Autodesk Inventor part; units mm, degrees
ref_plane "YZ Plane" through (0, 0, 0) normal (1, 0, 0) x (0, 1, 0)
ref_plane "XZ Plane" through (0, 0, 0) normal (0, 1, 0) x (-1, 0, 0)
ref_plane "XY Plane" through (0, 0, 0) normal (0, 0, 1) x (1, 0, 0)
sketch "スケッチ1" plane through (0, 0, 0) normal (0, 0, 1) x (1, 0, 0)
  line L0 (0, 0) -> (15, 0)
  line L1 (15, 0) -> (15, 15)
  line L2 (15, 15) -> (0, 15)
  line L3 (0, 15) -> (0, 0)
  line L4 (1, 1) -> (14, 1)
  line L5 (14, 1) -> (14, 14)
  line L6 (14, 14) -> (1, 14)
  line L7 (1, 14) -> (1, 1)
  dimension "d0" = 15
  dimension "d1" = 15
  dimension "d2" = 13
  dimension "d3" = 13
  dimension "d4" = 1
  dimension "d5" = 1
extrude "押し出し1" add sketch "スケッチ1" along normal blind 46
sketch "スケッチ2" plane through (15, 0, 0) normal (1, 0, 0) x (0, 0, -1)
  circle A0 centre (-5, 7.5) radius 1.6
  line L0 (0, 0) -> (-46, 0)
  line L1 (0, 0) -> (0, 15)
  circle A1 centre (-41, 7.5) radius 1.6
  line L2 (-46, 0) -> (-46, 15)
  dimension "d8" = 3.2
  dimension "d9" = 7.5
  dimension "d10" = 5
  dimension "d11" = 3.2
  dimension "d12" = 5
hole "穴1" at (15, 7.5, 41) at (15, 7.5, 5) direction (-1, 0, 0) diameter 3.2 depth 15
sketch "スケッチ3" plane through (0, 15, 0) normal (0, 1, 0) x (1, 0, 0)
  circle A0 centre (7.5, -15) radius 1.6
  line L0 (15, 0) -> (15, -46)
  line L1 (15, 0) -> (0, 0)
  circle A1 centre (7.5, -31) radius 1.6
  line L2 (15, -46) -> (0, -46)
  dimension "d20" = 3.2
  dimension "d21" = 7.5
  dimension "d22" = 15
  dimension "d23" = 3.2
  dimension "d24" = 15
hole "穴2" at (7.5, 15, 31) at (7.5, 15, 15) direction (0, -1, 0) diameter 3.2 depth 15
equation "\"BendRadius\" = Thickness"
equation "\"BendReliefWidth\" = Thickness"
equation "\"BendReliefDepth\" = 0.5 * Thickness"
equation "\"CornerReliefSize\" = 4 * Thickness"
equation "\"MinimumRemnant\" = 2 * Thickness"
equation "\"TransitionRadius\" = BendRadius"
equation "\"JacobiRadiusSize\" = BendRadius"
equation "\"GapSize\" = Thickness"
properties part number "nhk29"
Verification items for the finished model (mm, model axes). A direction names the side the tool comes from. Round coordinates to 2 decimals unless told otherwise and drop trailing zeros. Loops run counter-clockwise (first coordinate to the right, second up) from the corner with the lowest first, then second, coordinate; pieces in that order, holes last. Notation, with made-up numbers: (8.25, 18.25) - (66.25, 18.25) arc R24 cw to (66.25, 41.25) - close; hole circle Ø3 at (1.5, 21.25). An arc over 180 degrees is marked (long way). Write item = value, one per line.
Q1. Sectioned sample at B-B on y = 13.5. Record the boundary of the cut face in (x, z).
Here are the results:
outline = (0, 0) - (1, 0) - (1, 46) - (0, 46) - close; (14, 0) - (15, 0) - (15, 46) - (14, 46) - close
Q2. Depth check by flat-ended pin: pin 1 (4 mm diameter, centred on x = 11, z = 36.5, fed in from -Y). Enter the tip coordinate at first touch or a pass-through.
Here are the results:
pin_1 = 0
Q3. Sectioned sample at D-D on x = 7.5. Record the boundary of the cut face in (y, z), plus the area to 3 significant figures.
Here are the results:
outline = (0, 0) - (1, 0) - (1, 13.4) - (0, 13.4) - close; (0, 16.6) - (1, 16.6) - (1, 29.4) - (0, 29.4) - close; (0, 32.6) - (1, 32.6) - (1, 46) - (0, 46) - close; (14, 0) - (15, 0) - (15, 13.4) - (14, 13.4) - close; (14, 16.6) - (15, 16.6) - (15, 29.4) - (14, 29.4) - close; (14, 32.6) - (15, 32.6) - (15, 46) - (14, 46) - close
area = 79.2 mm^2
Q4. Material ranges on L1, parallel to Z at x = 7.5, y = 0.4; L2, parallel to X at y = 12.5, z = 7; L3, parallel to Y at x = 0.7, z = 41, recorded low to high.
Here are the results:
L1 = 0 to 13.4, 16.6 to 29.4, 32.6 to 46
L2 = 0 to 1, 14 to 15
L3 = 0 to 5.9, 9.1 to 15
Q5. Tool access check on faces 1 (the flat face through (1, 8, 23)), 2 (the cylindrical face through (8.47, 0.49, 29.73)). Record the directions out of +Z, -Z, +X, -X, +Y, -Y that give a thin tool (end or side, any length) a straight path to the whole face; none if there is none.
Here are the results:
face_1 = +Z, -Z
face_2 = +Y, -Y
Q6. Mould release check, pull along Z, two halves, no side actions. Record for faces 3 (the cylindrical face through (14.49, 9.06, 41.35)), 4 (the flat face through (0.7, 7.6, 0)), 5 (the flat face through (14, 7, 23)): +Z half, -Z half, draft (parallel to the pull), parting line (faces both ways), or undercut.
Here are the results:
face_3 = undercut
face_4 = -Z half
face_5 = draft
Q7. Sectioned sample at A-A on z = 41. Record the boundary of the cut face in (x, y), plus the area to 3 significant figures.
Here are the results:
outline = (0, 0) - (15, 0) - (15, 5.9) - (14, 5.9) - (14, 1) - (1, 1) - (1, 5.9) - (0, 5.9) - close; (0, 9.1) - (1, 9.1) - (1, 14) - (14, 14) - (14, 9.1) - (15, 9.1) - (15, 15) - (0, 15) - close
area = 49.6 mm^2
